Part model, mm, in its own coordinate system. A direction names the side the tool comes from. Give positions to 0.01 mm unless a question says otherwise; leave off trailing zeros. Write each loop counter-clockwise with the first axis right and the second up, starting at its lowest first coordinate (ties: lowest second). Pieces come first, ordered by that corner, then holes. Notation, with made-up numbers: M 13,49 L 52,49 A27 ccw 52,76 Z; hole C 5,0.5 d7. An arc over 180 degrees is marked long. Use a Markdown table: item, result.
```python
from build123d import *

# Parameters (mm, degrees)
F0_W     = 28
F0_H     = 7.4
F1_DEPTH = 22
F3_D     = 4.4
F4_W     = 26
F4_H     = 20
F5_DEPTH = 25
F7_D     = 4.4


# Not quite as in the source:
# - a feature of the source that left no trace in its solid (it failed there, or was rolled back) is left out
# - a feature names something its author has since deleted; it is built from what else it names


with BuildPart() as f1:
    # F0 (on Top) → F1 (new body)
    with BuildSketch(Plane.XY):
        with Locations((-14, -3.7)):
            Rectangle(F0_W, F0_H)
    extrude(amount=F1_DEPTH)

    # F3 (through all)
    with Locations(Plane.XY.offset(22)):
        with Locations((-24, -3.7), (-8, -3.7)):
            Hole(F3_D / 2)

    # F4 (on face) → F5 (cut)
    with BuildSketch(Plane(origin=(0, 0, 0), x_dir=(-1, 0, 0), z_dir=(0, 1, 0))):
        with Locations((15, 12)):
            Rectangle(F4_W, F4_H)
    extrude(amount=-F5_DEPTH, mode=Mode.SUBTRACT)

    # F7 (through all)
    with Locations(Plane(origin=(-2, 0, 0), x_dir=(0, -1, 0), z_dir=(-1, 0, 0))):
        with Locations((3.7, 16.2), (3.7, 6.2)):
            Hole(F7_D / 2)


solid = f1.part
```
1. Two-plate mould, pull along X, no slides. Class faces 3 (the cylindrical face through (-26.032, -4.543, 0.986)), 4 (the cylindrical face through (-0.986, -4.177, 14.052)), 5 (the flat face through (-2, -4, 12)): released by +X, released by -X, zero draft, split by the parting line, or undercut.
Findings below:
| item | result |
|---|---|
| face 3 | undercut |
| face 4 | zero draft |
| face 5 | released by -X |
2. Cut at A-A, the plane x = -8. Give the cut face in (y, z), then the cut area to 3 significant figures.
Findings below:
| item | result |
|---|---|
| outline | M -7.4,0 L -5.9,0 L -5.9,2 L -7.4,2 Z; M -1.5,0 L 0,0 L 0,2 L -1.5,2 Z |
| area | 6.00 mm2 |
3. Cut at C-C, the plane z = 6.2. Give the cut face in (x, y), then the cut area to 3 significant figures.
Findings below:
| item | result |
|---|---|
| outline | M -2,-7.4 L 0,-7.4 L 0,-5.9 L -2,-5.9 Z; M -2,-1.5 L 0,-1.5 L 0,0 L -2,0 Z |
| area | 6.00 mm2 |
4. Tool access for faces 1 (the flat face through (-15, -4, 2)), 2 (the flat face through (-8, 0, 1)): list every direction of +Z, -Z, +X, -X, +Y, -Y with a clear straight run to the whole face (end or side of a thin tool).
Findings below:
| item | result |
|---|---|
| face 1 | +Z, -X, +Y, -Y |
| face 2 | +Z, -Z, +X, -X, +Y |
5. Drop flat-ended pins along their axis: P1, Ø3.5, axis at x = -17, y = -2.5, coming from the +Z side; P2, Ø4, axis at y = -2, z = 13.5, coming from the -X side. Give the stop position or say it passes through.
Findings below:
| item | result |
|---|---|
| P1 | z = 2 |
| P2 | x = -2 |
6. Drill centre lines: L1, parallel to Z at x = -1.2, y = -3.7; L2, parallel to Y at x = -8, z = 0.95; L3, parallel to Z at x = -10.75, y = -4.5. Where is each one in solid material? Low to high.
Findings below:
| item | result |
|---|---|
| L1 | 0 to 4, 8.4 to 14, 18.4 to 22 |
| L2 | -7.4 to -5.9, -1.5 to 0 |
| L3 | 0 to 2 |
7. Cut at D-D, the plane y = -1. Give the cut face in (x, z).
Findings below:
| item | result |
|---|---|
| outline | M -28,0 L 0,0 L 0,22 L -2,22 L -2,2 L -28,2 Z |
8. Cut at B-B, the plane y = -3.7. Give the cut face in (x, z).
Findings below:
| item | result |
|---|---|
| outline | M -28,0 L -26.2,0 L -26.2,2 L -28,2 Z; M -21.8,0 L -10.2,0 L -10.2,2 L -21.8,2 Z; M -5.8,0 L 0,0 L 0,4 L -2,4 L -2,2 L -5.8,2 Z; M -2,8.4 L 0,8.4 L 0,14 L -2,14 Z; M -2,18.4 L 0,18.4 L 0,22 L -2,22 Z |
